```python
from build123d import *

# Parameters (mm, degrees)
SKETCH1_W                 = 42
SKETCH1_H                 = 127
BOSS_EXTRUDE1_DEPTH       = 5.1
SKETCH2_W                 = 40
SKETCH2_H                 = 6
CUT_EXTRUDE1_DEPTH        = 8.7
SKETCH3_W                 = 15
SKETCH3_H                 = 2
BOSS_EXTRUDE2_DEPTH       = 0.5
TAB_PROFILE_W             = 10.5
TAB_PROFILE_H             = 0.5
FILLET2_R                 = 0.75
FILLET1_R                 = 1.25
FILLET4_R                 = 0.75
FILLET3_R                 = 1.25
F_6_CLEARANCE_HOLE1_D     = 3.6576
F_6_CLEARANCE_HOLE1_DEPTH = 0.5
F_6_CLEARANCE_HOLE2_D     = 3.6576
F_6_CLEARANCE_HOLE2_DEPTH = 0.5


with BuildPart() as part:
    # Sketch1 → Boss-Extrude1 (new, symmetric)
    with BuildSketch(Plane.XY):
        with Locations((0, 63.5)):
            Rectangle(SKETCH1_W, SKETCH1_H)
    extrude(amount=BOSS_EXTRUDE1_DEPTH, both=True)

    # Sketch2 → Cut-Extrude1 (cut)
    with BuildSketch(Plane.XY.offset(5.1)):
        with Locations((0, 124)):
            Rectangle(SKETCH2_W, SKETCH2_H)
    extrude(amount=-CUT_EXTRUDE1_DEPTH, mode=Mode.SUBTRACT)

    # Sketch3 → Boss-Extrude2 (add, symmetric)
    with BuildSketch(Plane(origin=(0, 0, -4.6), x_dir=(-1, 0, 0), z_dir=(0, 0, -1))):
        with Locations((-10.5, 128)):
            Rectangle(SKETCH3_W, SKETCH3_H)
        with Locations((10.5, 128)):
            Rectangle(SKETCH3_W, SKETCH3_H)
    extrude(amount=BOSS_EXTRUDE2_DEPTH, both=True)

    # Tabs: sweep along a path in Tab Bend
    with BuildLine(Plane(origin=(0, 0, 0), x_dir=(0, 0, -1), z_dir=(1, 0, 0))) as tabs_path:
        Line((4.6, 129), (4.6, 135))
        Line((4.6, 135), (-4.6, 135))
    # Tab Profile → Tabs (sweep)
    with BuildSketch(Plane(origin=(0, 129, 0), x_dir=(1, 0, 0), z_dir=(0, 1, 0))):
        with Locations((-10.5, 4.6)):
            Rectangle(TAB_PROFILE_W, TAB_PROFILE_H)
        with Locations((10.5, 4.6)):
            Rectangle(TAB_PROFILE_W, TAB_PROFILE_H)
    sweep(path=tabs_path.line, transition=Transition.RIGHT)

    # Fillet2
    fillet2_edges = [part.edges().sort_by_distance(p)[0] for p in [
        (10.5, 134.75, -4.35),
    ]]
    fillet(fillet2_edges, radius=FILLET2_R)

    # Fillet1
    fillet1_edges = [part.edges().sort_by_distance(p)[0] for p in [
        (10.5, 135.25, -4.85),
    ]]
    fillet(fillet1_edges, radius=FILLET1_R)

    # Fillet4
    fillet4_edges = [part.edges().sort_by_distance(p)[0] for p in [
        (-10.5, 134.75, -4.35),
    ]]
    fillet(fillet4_edges, radius=FILLET4_R)

    # Fillet3
    fillet3_edges = [part.edges().sort_by_distance(p)[0] for p in [
        (-10.5, 135.25, -4.85),
    ]]
    fillet(fillet3_edges, radius=FILLET3_R)

    # #6 Clearance Hole1
    with Locations(Plane(origin=(0, 135.25, 0), x_dir=(1, 0, 0), z_dir=(0, 1, 0))):
        with Locations((-10.5, -1)):
            Hole(F_6_CLEARANCE_HOLE1_D / 2, depth=F_6_CLEARANCE_HOLE1_DEPTH)

    # #6 Clearance Hole2
    with Locations(Plane(origin=(0, 135.25, 0), x_dir=(1, 0, 0), z_dir=(0, 1, 0))):
        with Locations((10.5, -1)):
            Hole(F_6_CLEARANCE_HOLE2_D / 2, depth=F_6_CLEARANCE_HOLE2_DEPTH)


solid = part.part
```
Work out the finished part from the listing and answer in its coordinate system (mm). A direction names the side the tool comes from. Round coordinates to 2 decimals unless told otherwise and drop trailing zeros. Write each loop counter-clockwise with the first axis right and the second up, starting at its lowest first coordinate (ties: lowest second). Pieces come first, ordered by that corner, then holes. Notation, with made-up numbers: (33, -34.75) -> (78, -34.75) arc R31 ccw to (78, -4.75) -> close; hole circle Ø8 at (67.5, 84). An arc over 180 degrees is marked (long way). Write each question's results on one line, items separated by ' | '.
1) The part is cut by section C-C (x = -1). Write down the section's boundary in (y, z), and give its area (3 significant figures).
Findings:
outline: (0, -5.1) -> (127, -5.1) -> (127, -3.6) -> (121, -3.6) -> (121, 5.1) -> (0, 5.1) -> close | area: 1,240 mm²
2) Flat-ended cylindrical pins translate along their axes: pin 1 (5.5 mm diameter, centred on x = 10, y = 131, fed in from +Z); pin 2 (2 mm diameter, centred on x = 11.5, y = 127.5, fed in from +Z); pin 3 (3 mm diameter, centred on y = 131.5, z = 1, fed in from -X); pin 4 (1.5 mm diameter, centred on x = 0.5, z = 2.5, fed in from +Y). Find the tip coordinate at first contact, or state that the pin passes through.
Findings:
pin 1: stops at z = -4.1 | pin 2: stops at z = -3.6 | pin 3: passes through | pin 4: stops at y = 121
3) Which of the six approach directions +Z, -Z, +X, -X, +Y, -Y give full straight-line access (tool end or side, diameter ignored) to faces 5 (the flat face through (20, 124, 1)), 6 (the cylindrical face through (11.951, 134.996, 2.113)), 7 (the flat face through (0, 124, -3.6)), 8 (the flat face through (10, 134.75, -1)), 9 (the flat face through (5.25, 135, -2))?
Findings:
face 5: +Z, +Y | face 6: +Y | face 7: +Z | face 8: +Z, +X, -X | face 9: +Z, -Z, +Y
4) The part is cut by section B-B (x = 10.5). Write down the section's boundary in (y, z), and give its area (3 significant figures).
Findings:
outline: (0, -5.1) -> (129, -5.1) -> (129, -4.85) -> (134, -4.85) arc R1.25 ccw to (135.25, -3.6) -> (135.25, -0.83) -> (134.75, -0.83) -> (134.75, -3.6) arc R0.75 cw to (134, -4.35) -> (129, -4.35) -> (129, -4.1) -> (127, -4.1) -> (127, -3.6) -> (121, -3.6) -> (121, 5.1) -> (0, 5.1) -> close; (134.75, 2.83) -> (135.25, 2.83) -> (135.25, 4.6) -> (134.75, 4.6) -> close | area: 1,250 mm²
5) Consider line 1 along Y through (x, z) = (-13.5, -3.25); line 2 along Y through (x, z) = (19.5, -3.5); line 3 along Z through (x, y) = (-10.5, 135.05). Determine where each line is inside the solid, lowest interval first. Write a range as [from, to].
Findings:
line 1: y = [0, 121], [134.75, 135.25] | line 2: y = [0, 121] | line 3: z = [-4.28, -0.83], [2.83, 4.6]
6) For a pull along X with two mould halves and no side action, classify faces 1 (the flat face through (0, 121, 1)), 2 (the flat face through (11, 132, -4.85)), 3 (the flat face through (-15.75, 135, -2)), 4 (the flat face through (15.75, 135, -2)) as +X half, -X half, draft (parallel to the pull), parting line (faces both ways), or undercut.
Findings:
face 1: undercut | face 2: draft | face 3: -X half | face 4: +X half
7) The part is cut by section A-A (z = 1). Write down the section's boundary in (x, y), and give its area (3 significant figures).
Findings:
outline: (-21, 0) -> (21, 0) -> (21, 127) -> (20, 127) -> (20, 121) -> (-20, 121) -> (-20, 127) -> (-21, 127) -> close; (-15.75, 134.75) -> (-12.33, 134.75) -> (-12.33, 135.25) -> (-15.75, 135.25) -> close; (-8.67, 134.75) -> (-5.25, 134.75) -> (-5.25, 135.25) -> (-8.67, 135.25) -> close; (5.25, 134.75) -> (8.67, 134.75) -> (8.67, 135.25) -> (5.25, 135.25) -> close; (12.33, 134.75) -> (15.75, 134.75) -> (15.75, 135.25) -> (12.33, 135.25) -> close | area: 5,100 mm²
